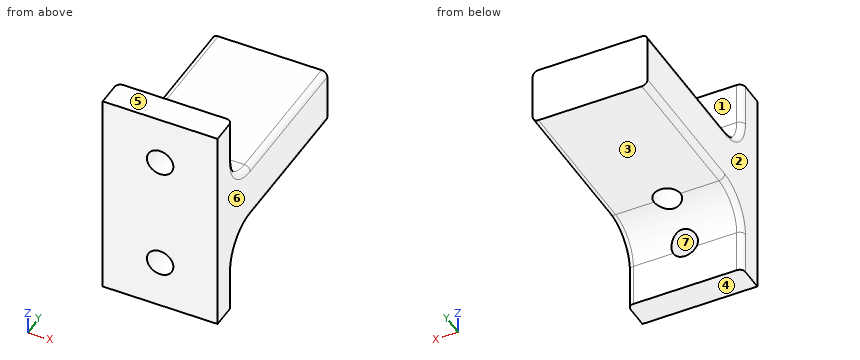
from build123d import *

# Parameters (mm, degrees)
BOSS_EXTRUDE1_DEPTH     = 25.4
FILLET1_R               = 7.62
SKETCH2_R               = 2.921
CUT_EXTRUDE1_DEPTH      = 59.354392508
FILLET2_R               = 1.27
CUT_EXTRUDE2_DEPTH      = 62.187777579
CUT_EXTRUDE2_DEPTH_BACK = 62.187777579
SKETCH3_R               = 2.921


with BuildPart() as part:
    # Sketch1 → Boss-Extrude1 (new body)
    with BuildSketch(Plane(origin=(0, 0, 0), x_dir=(0, 0, -1), z_dir=(1, 0, 0))):
        Polygon((-6.35, 46.99), (6.35, 46.99), (6.35, 6.35), (23.495, 6.35), (23.495, 0), (-23.495, 0), (-23.495, 6.35), (-6.35, 6.35), align=None)
    extrude(amount=BOSS_EXTRUDE1_DEPTH)

    # Fillet1
    fillet1_edges = [part.edges().sort_by_distance(p)[0] for p in [
        (12.7, 6.35, -6.35),
        (12.7, 6.35, 6.35),
    ]]
    fillet(fillet1_edges, radius=FILLET1_R)

    # Sketch2 → Cut-Extrude1 (cut, through all)
    with BuildSketch(Plane.XZ):
        with Locations(Location((12.7, 12.7, 0), (0, 0, 270))):
            Circle(SKETCH2_R)
        with Locations(Location((12.7, -12.7, 0), (0, 0, 334.228538259))):
            Circle(SKETCH2_R)
    extrude(amount=-CUT_EXTRUDE1_DEPTH, mode=Mode.SUBTRACT)

    # Fillet2
    fillet2_edges = [part.edges().sort_by_distance(p)[0] for p in [
        (0, 30.48, 6.35),
        (25.4, 30.48, 6.35),
        (0, 6.35, 18.7325),
        (25.4, 6.35, 18.7325),
        (0, 30.48, -6.35),
        (25.4, 30.48, -6.35),
        (0, 8.581846327, 8.581846327),
        (25.4, 8.581846327, 8.581846327),
        (0, 8.581846327, -8.581846327),
        (25.4, 8.581846327, -8.581846327),
        (25.4, 6.35, -18.7325),
        (0, 6.35, -18.7325),
    ]]
    fillet(fillet2_edges, radius=FILLET2_R)

    # Sketch3 → Cut-Extrude2 (cut, two sides: drawn at the far end of the back side and taken through both)
    with BuildSketch(Plane(origin=(0, 0, -6.35), x_dir=(-1, 0, 0), z_dir=(0, 0, -1)).offset(-CUT_EXTRUDE2_DEPTH_BACK)):
        with Locations((-12.7, 13.97)):
            Circle(SKETCH3_R)
    extrude(amount=CUT_EXTRUDE2_DEPTH + CUT_EXTRUDE2_DEPTH_BACK, mode=Mode.SUBTRACT)


solid = part.part
Can you work these out from the model? Positions are in its coordinate system, mm. Face numbers are marked on the shaded views. A direction names the side the tool comes from. Coordinates: 2 decimals unless noted, no trailing zeros. Order: outer loops, then holes, each group sorted by start corner. A loop starts at its lowest first (then second) coordinate and runs counter-clockwise, first axis right, second up. Notation, with made-up numbers: (87, 9.25) - (97, 9.25) arc R22 cw to (97, 29.25) - close; hole circle Ø11 at (-19, 80). An arc over 180 degrees is marked (long way). Answer as a JSON object with one key per item and string values. Group by question number.
Q1. I need wall thicknesses on line 1 (Z direction, x = 12.7, y = 2.5) (3 decimals); line 2 (X direction, y = 2.5, z = 12.7); line 3 (Y direction, x = 12.7, z = -2.25). Which ranges of each line are inside material? Lowest first, please. Write a range as from..to.
Q2. Imagine slicing it at D-D (x = 23.25). Please give me the cut outline in (y, z) (3 decimals).
Q3. Imagine slicing it at C-C (y = 40.5). Please give me the cut outline in (x, z).
Q4. On a 3-axis mill with a long thin cutter (end or side, diameter ignored), from which of +Z, -Z, +X, -X, +Y, -Y can I reach the whole of each face in a straight line? I mean the marked faces 1, 2 and 3. Say none if no direction works.
Q5. Imagine slicing it at B-B (z = 3.5). Please give me the cut outline in (x, y).
Q6. We'd pull the mould along Z, two halves only. Please class the marked faces 4, 5, 6 and 7: +Z half, -Z half, draft (parallel to the pull), parting line (faces both ways), or undercut.
Q7. Imagine slicing it at A-A (x = 12.7). Please give me the cut outline in (y, z) (3 decimals).
Q8. Will these pins go through, and if not, where does the flat tip stop? P1, Ø3, axis at x = 10.5, z = 1, coming from the -Y side; P2, Ø6.5, axis at x = 12.7, z = -12.7, coming from the +Y side; P3, Ø4, axis at x = 9, y = 9, coming from the -Z side; P4, Ø9.5, axis at x = 12.7, y = 13.97, coming from the -Z side.
Determined:
{
 "1": {"line 1": "z = -23.495..-15.621, -9.779..9.779, 15.621..23.495", "line 2": "x = 0..9.78, 15.62..25.4", "line 3": "y = 0..11.05, 16.89..46.99"},
 "2": {"outline": "(0, -23.495) - (6.35, -23.495) - (6.35, -13.97) arc R7.62 cw to (13.97, -6.35) - (46.99, -6.35) - (46.99, 6.35) - (13.97, 6.35) arc R7.62 cw to (6.35, 13.97) - (6.35, 23.495) - (0, 23.495) - close"},
 "3": {"outline": "(0, -5.08) arc R1.27 ccw to (1.27, -6.35) - (24.13, -6.35) arc R1.27 ccw to (25.4, -5.08) - (25.4, 5.08) arc R1.27 ccw to (24.13, 6.35) - (1.27, 6.35) arc R1.27 ccw to (0, 5.08) - close"},
 "4": {"face 1": "+Z, +X, -X, +Y", "face 2": "+Z, -Z, -X, +Y, -Y", "face 3": "-Z, +X, -X, +Y"},
 "5": {"outline": "(0, 0) - (25.4, 0) - (25.4, 46.99) - (0, 46.99) - close; hole circle Ø5.84 at (12.7, 13.97)"},
 "6": {"face 4": "-Z half", "face 5": "+Z half", "face 6": "draft", "face 7": "undercut"},
 "7": {"outline": "(0, -23.495) - (6.35, -23.495) - (6.35, -15.621) - (0, -15.621) - close; (0, -9.779) - (7.606, -9.779) arc R7.62 cw to (11.049, -6.932) - (11.049, 6.932) arc R7.62 cw to (7.606, 9.779) - (0, 9.779) - close; (0, 15.621) - (6.35, 15.621) - (6.35, 23.495) - (0, 23.495) - close; (16.891, -6.35) - (46.99, -6.35) - (46.99, 6.35) - (16.891, 6.35) - close"},
 "8": {"P1": "stops at y = 0", "P2": "stops at y = 7.84", "P3": "stops at z = -10.89", "P4": "stops at z = -8.01"}
}
